from build123d import *

# Parameters (mm, degrees)
SKETCH1_W           = 20.8
SKETCH1_H           = 14.3
SKETCH1_W_2         = 16.8
SKETCH1_H_2         = 10.3
BOSS_EXTRUDE1_DEPTH = 12.5
SKETCH2_W           = 20.8
SKETCH2_H           = 14.3
BOSS_EXTRUDE2_DEPTH = 1
SKETCH3_R           = 5.85
CUT_EXTRUDE2_DEPTH  = 2
BOSS_EXTRUDE3_DEPTH = 6
CUT_EXTRUDE3_DEPTH  = 14.3


with BuildPart() as part:
    # Sketch1 → Boss-Extrude1 (new body)
    with BuildSketch(Plane(origin=(0, 0, 0), x_dir=(1, 0, 0), z_dir=(0, 1, 0))):
        Rectangle(SKETCH1_W, SKETCH1_H)
        Rectangle(SKETCH1_W_2, SKETCH1_H_2, mode=Mode.SUBTRACT)
    extrude(amount=BOSS_EXTRUDE1_DEPTH)

    # Sketch2 → Boss-Extrude2 (add)
    with BuildSketch(Plane.XZ):
        Rectangle(SKETCH2_W, SKETCH2_H)
    extrude(amount=BOSS_EXTRUDE2_DEPTH)

    # Sketch3 → Cut-Extrude2 (cut)
    with BuildSketch(Plane.ZY.offset(10.4)):
        with Locations((0, 5.25)):
            Circle(SKETCH3_R)
    extrude(amount=-CUT_EXTRUDE2_DEPTH, mode=Mode.SUBTRACT)

    # Sketch4 → Boss-Extrude3 (add, symmetric)
    with BuildSketch(Plane.XY):
        Polygon((8.4, 11.5), (1.760471904, 0), (8.4, 0), align=None)
    extrude(amount=BOSS_EXTRUDE3_DEPTH, both=True)

    # Sketch5 → Cut-Extrude3 (cut)
    with BuildSketch(Plane.XY.offset(7.15)):
        Polygon((10.4, -1), (10.4, 11.5), (3.183121635, -1), align=None)
    extrude(amount=-CUT_EXTRUDE3_DEPTH, mode=Mode.SUBTRACT)


solid = part.part
Model file for the job. Use its own axes, mm. A direction names the side the tool comes from. Round coordinates to 2 decimals unless told otherwise and drop trailing zeros. Loops run counter-clockwise (first coordinate to the right, second up) from the corner with the lowest first, then second, coordinate; pieces in that order, holes last.
1. Band-saw the part on B-B, the plane x = 1.25. List the corners of the cut face in (y, z).
Check values:
outline: (-1, -7.15) - (12.5, -7.15) - (12.5, -5.15) - (0, -5.15) - (0, 5.15) - (12.5, 5.15) - (12.5, 7.15) - (-1, 7.15) - close
2. Tool access for faces 1 (the flat face through (-2, 6, -7.15)), 2 (the flat face through (-2, 6, 5.15)): list every direction of +Z, -Z, +X, -X, +Y, -Y with a clear straight run to the whole face (end or side of a thin tool).
Check values:
face 1: -Z, +X, -X, +Y, -Y
face 2: +Y
3. Band-saw the part on D-D, the plane z = -2.25. List the corners of the cut face in (x, y), and give its area (3 significant figures).
Check values:
outline: (-10.4, -1) - (3.18, -1) - (10.4, 11.5) - (10.4, 12.5) - (8.4, 12.5) - (8.4, 11.5) - (1.76, 0) - (-8.4, 0) - (-8.4, -0.15) - (-10.4, -0.15) - close; (-10.4, 10.65) - (-8.4, 10.65) - (-8.4, 12.5) - (-10.4, 12.5) - close
area: 42.3 mm2
4. Band-saw the part on A-A, the plane z = 0. List the corners of the cut face in (x, y).
Check values:
outline: (-10.4, -1) - (3.18, -1) - (10.4, 11.5) - (10.4, 12.5) - (8.4, 12.5) - (8.4, 11.5) - (1.76, 0) - (-8.4, 0) - (-8.4, -0.6) - (-10.4, -0.6) - close; (-10.4, 11.1) - (-8.4, 11.1) - (-8.4, 12.5) - (-10.4, 12.5) - close
5. Mould opens along Y. For faces 3 (the cylindrical face through (-9.41, 7.01, 5.58)), 4 (the flat face through (-8.4, 0.7, -4.4)), 5 (the flat face through (-4, -1, 0)) say: +Y half, -Y half, draft (parallel to the pull), parting line (faces both ways), or undercut.
Check values:
face 3: undercut
face 4: draft
face 5: -Y half
6. Drop flat-ended pins along their axis: P1, Ø3, axis at x = -3.5, z = -0.5, coming from the +Y side; P2, Ø1.5, axis at y = 7, z = -2, coming from the -X side; P3, Ø2, axis at y = 0.5, z = 3.5, coming from the +X side. Give the stop position or say it passes through.
Check values:
P1: stops at y = 0
P2: stops at x = 5.37
P3: stops at x = 4.63
7. Band-saw the part on C-C, the plane y = 1.25. List the corners of the cut face in (x, z).
Check values:
outline: (-10.4, -7.15) - (4.48, -7.15) - (4.48, 7.15) - (-10.4, 7.15) - (-10.4, 4.27) - (-8.4, 4.27) - (-8.4, 5.15) - (2.48, 5.15) - (2.48, -5.15) - (-8.4, -5.15) - (-8.4, -4.27) - (-10.4, -4.27) - close
8. Wall check: probe 1 along Y at (x, z) = (-9.3, 0); probe 2 along Z at (x, y) = (-9.8, 5.25); probe 3 along Z at (x, y) = (-3, 7.75). Give the ranges that are in metal, low to high.
Check values:
probe 1: y = -1 to -0.6, 11.1 to 12.5
probe 2: z = -7.15 to -5.85, 5.85 to 7.15
probe 3: z = -7.15 to -5.15, 5.15 to 7.15
